from build123d import *

# Parameters (mm, degrees)
F0_R     = 8
F1_DEPTH = 4
F2_W     = 1800
F2_H     = 5
F3_DEPTH = 50
F4_R     = 8
F5_DEPTH = 25


with BuildPart() as f1:
    # F0 (on Front) → F1 (new body)
    with BuildSketch(Plane.XZ):
        Polygon((-1800, 0), (0, 0), (0, 1600), (-2410, 1600), (-1800, 990), (-1800, 870), (-2015, 530), (-1800, 530), align=None)
        with Locations((-1880, 1112.426407)):
            Circle(F0_R, mode=Mode.SUBTRACT)
        with Locations((-1986.066017, 1218.492424)):
            Circle(F0_R, mode=Mode.SUBTRACT)
        with Locations((-2092.132034, 1324.558441)):
            Circle(F0_R, mode=Mode.SUBTRACT)
        with Locations((-2198.198052, 1430.624458)):
            Circle(F0_R, mode=Mode.SUBTRACT)
        with Locations((-2304.264069, 1536.690476)):
            Circle(F0_R, mode=Mode.SUBTRACT)
    extrude(amount=F1_DEPTH)

    # F2 (on face) → F3 (join)
    with BuildSketch(Plane(origin=(0, 0, 0), x_dir=(-1, 0, 0), z_dir=(0, 1, 0))):
        with Locations((900, 2.5)):
            Rectangle(F2_W, F2_H)
    extrude(amount=F3_DEPTH)

    # F4 (on face) → F5 (cut)
    with BuildSketch(Plane.XY.offset(5)):
        with Locations((-50, 25)):
            Circle(F4_R)
        with Locations((-550, 25)):
            Circle(F4_R)
        with Locations((-1050, 25)):
            Circle(F4_R)
        with Locations((-1550, 25)):
            Circle(F4_R)
        with Locations((-1750, 25)):
            Circle(F4_R)
    extrude(amount=-F5_DEPTH, mode=Mode.SUBTRACT)


solid = f1.part
Could you check a few things on this model? Use its own coordinates, in mm. A direction names the side the tool comes from. Coordinates: 2 decimals unless noted, no trailing zeros. Write each loop counter-clockwise with the first axis right and the second up, starting at its lowest first coordinate (ties: lowest second). Pieces come first, ordered by that corner, then holes. Notation, with made-up numbers: M 64.25,61 L 91.25,61 A15 cw 91.25,88 Z; hole C -22,51 d8. An arc over 180 degrees is marked long. One line per question, with ' | ' between items.
1) If we mould it in two halves opening along Z, with no side actions, what happens to faces 1 (the face through (-887, 23, 0)), 2 (the face through (-954, -4, 811)), 3 (the face through (-1905.995, -1.972, 702.38))? For each: released by +Z, released by -Z, zero draft, split by the parting line, or undercut.
Checks:
face 1: released by -Z | face 2: zero draft | face 3: undercut
2) For faces 4 (the face through (0, -3, 796)), 5 (the face through (-887, 25, 5)), 6 (the face through (-1800, -3, 264)), 7 (the face through (-2109, -2, 1299)), which set-ups out of +Z, -Z, +X, -X, +Y, -Y let a thin tool reach every point of the face, with its end or its side?
Checks:
face 4: +Z, -Z, +X, +Y, -Y | face 5: +Z, +X, -X, +Y | face 6: -Z, -X, +Y, -Y | face 7: -X, +Y, -Y
3) I need wall thicknesses on probe 1 along Y at (x, z) = (-50, 3); probe 2 along Y at (x, z) = (-1640.5, 109); probe 3 along Z at (x, y) = (-729, 28). Which ranges of each line are inside material? Lowest first, please. Write a range as [from, to].
Checks:
probe 1: [-4, 17], [33, 50] | probe 2: [-4, 0] | probe 3: [0, 5]
4) Imagine slicing it at A-A, the plane x = -321.5. Write out the boundary of the cut face in (y, z).
Checks:
outline: M -4,0 L 50,0 L 50,5 L 0,5 L 0,1600 L -4,1600 Z
5) For pin 1 Ø8 at (x, y) = (-800, 36) entering from +Z; pin 2 Ø2 at (x, y) = (-1887.5, -2) entering from -Z; pin 3 Ø1.5 at (x, z) = (-1553, 832.5) entering from +Y, each with a flat end and sliding along its axis, tell me the tip position at first contact or that it passes through.
Checks:
pin 1: z = 5 | pin 2: z = 530 | pin 3: y = 0
6) Imagine slicing it at C-C, the plane z = 933.5. Write out the boundary of the cut face in (x, y), and give its area (3 significant figures).
Checks:
outline: M -1800,-4 L 0,-4 L 0,0 L -1800,0 Z | area: 7,200 mm²
7) Imagine slicing it at B-B, the plane z = 1373.5. Write out the boundary of the cut face in (x, y).
Checks:
outline: M -2183.5,-4 L 0,-4 L 0,0 L -2183.5,0 Z
